The model under review builds one solid part; all positions refer to its coordinate system, in mm. Face numbers are marked on the shaded views. Coordinates: 2 decimals unless noted, no trailing zeros. Loops run counter-clockwise (first coordinate to the right, second up) from the corner with the lowest first, then second, coordinate; pieces in that order, holes last. Notation, with made-up numbers: M 73.5,78 L 117.5,78 A28 ccw 117.5,99 Z; hole C 38.25,29.25 d11. An arc over 180 degrees is marked long. Write item = value, one per line. Start each with the question number.
Q1. We need section B-B on x = 118.5. Give the boundary of the cut face in (y, z), and give its area (3 significant figures).
Q2. Wall thickness on probe 1 along X at (y, z) = (13.25, 1.35); probe 2 along Y at (x, z) = (54, 1.4): over which ranges is each line inside the solid? List them lowest first.
Q3. We need section A-A on z = 0.7. Give the boundary of the cut face in (x, y), and give its area (3 significant figures).
Q4. Mouldability with a two-part tool opening along Z and no side actions: class the marked faces 1 and 2 as released by +Z, released by -Z, zero draft, split by the parting line, or undercut.
from build123d import *

# Parameters (mm, degrees)
BOSS_EXTRUDE1_DEPTH = 2


with BuildPart() as part:
    # Sketch1 → Boss-Extrude1 (new body)
    with BuildSketch(Plane.XY):
        Polygon((0, 0), (0, -15), (23, -15), (23, -13), (123, -13), (123, -15), (146, -15), (146, 0), align=None)
    boss_extrude1 = extrude(amount=BOSS_EXTRUDE1_DEPTH)

    # Mirror3: Boss-Extrude1 across plane
    add(boss_extrude1.mirror(Plane(origin=(0, 0, 2), x_dir=(0, 0, 1), z_dir=(0, -1, 0))))


solid = part.part
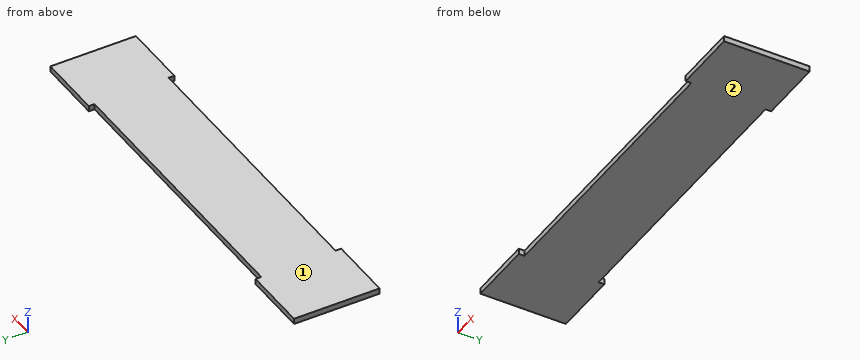
Returned:
q1.outline = M -13,0 L 13,0 L 13,2 L -13,2 Z
q1.area = 52.0 mm^2
q2.probe_1 = 0 to 23, 123 to 146
q2.probe_2 = -13 to 13
q3.outline = M 0,-15 L 23,-15 L 23,-13 L 123,-13 L 123,-15 L 146,-15 L 146,15 L 123,15 L 123,13 L 23,13 L 23,15 L 0,15 Z
q3.area = 3,980 mm^2
q4.face_1 = released by +Z
q4.face_2 = released by -Z
